Source: three-view drawing plus pictorial views. Frame: mm from the lowest corner of the part. A direction names the side the tool comes from. Coordinates: 2 decimals unless noted, no trailing zeros. Order: outer loops, then holes, each group sorted by start corner. A loop starts at its lowest first (then second) coordinate and runs counter-clockwise, first axis right, second up. Notation, with made-up numbers: M 33,-12.75 L 86,-12.75 A17 cw 86,-6.75 Z; hole C 0,60.5 d8. An arc over 180 degrees is marked long. One line per question, with ' | ' between items.
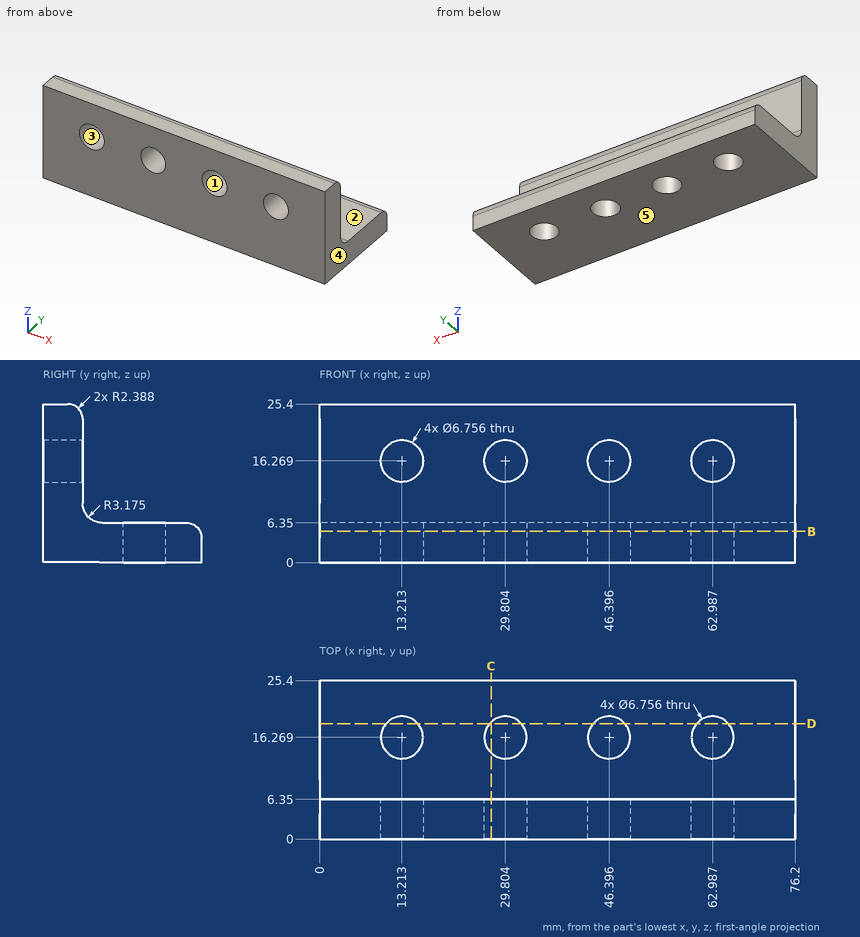
1. Material intervals for line 1 (X direction, y = 17.25, z = 5.25) (1 decimal); line 2 (Z direction, x = 17, y = 23), sorted ascending. Write a range as [from, to].
Response values:
line 1: x = [0, 10], [16.4, 26.6], [33, 43.2], [49.6, 59.8], [66.2, 76.2] | line 2: z = [0, 6.35]
2. Section B-B, the plane z = 5. Output: boundary loops of the cut face in (x, y) (1 decimal).
Response values:
outline: M 0,0 L 76.2,0 L 76.2,25.2 L 0,25.2 Z; hole C 13.2,16.3 d6.8; hole C 29.8,16.3 d6.8; hole C 46.4,16.3 d6.8; hole C 63,16.3 d6.8
3. Draft query along X for the marked faces 3, 4 and 5. Return one class per face: pulls with the +X half, pulls with the -X half, needs draft (parallel to the pull), parting line crosses it, or undercut.
Response values:
face 3: undercut | face 4: pulls with the +X half | face 5: needs draft
4. Pin query (flat end, axial travel): P1, Ø4, axis at x = 21, y = 13, coming from the +Z side; P2, Ø8, axis at x = 24, y = 9.5, coming from the +Z side; P3, Ø4, axis at x = 58.5, z = 19.5, coming from the +Y side. Return the tip coordinate at first contact, or that it passes through.
Response values:
P1: stops at z = 6.35 | P2: stops at z = 24.84 | P3: stops at y = 6.35
5. Section C-C, the plane x = 27.5. Give the number of separate pieces and of enclosed holes in the cut face, and give its area (3 significant figures).
Response values:
separate pieces: 3 | enclosed holes: 0 | area: 219 mm^2
6. Section D-D, the plane y = 18.5. Output: boundary loops of the cut face in (x, z).
Response values:
outline: M 0,0 L 10.68,0 L 10.68,6.35 L 0,6.35 Z; M 15.75,0 L 27.27,0 L 27.27,6.35 L 15.75,6.35 Z; M 32.34,0 L 43.86,0 L 43.86,6.35 L 32.34,6.35 Z; M 48.93,0 L 60.45,0 L 60.45,6.35 L 48.93,6.35 Z; M 65.52,0 L 76.2,0 L 76.2,6.35 L 65.52,6.35 Z
7. Access query for the marked faces 1 and 2. Directions: +Z, -Z, +X, -X, +Y, -Y. A direction counts if a zero-diameter tool reaches every point of the face in a straight line with its end or side. Return the directions, or none.
Response values:
face 1: +Y, -Y | face 2: +Z, +X, -X, +Y
